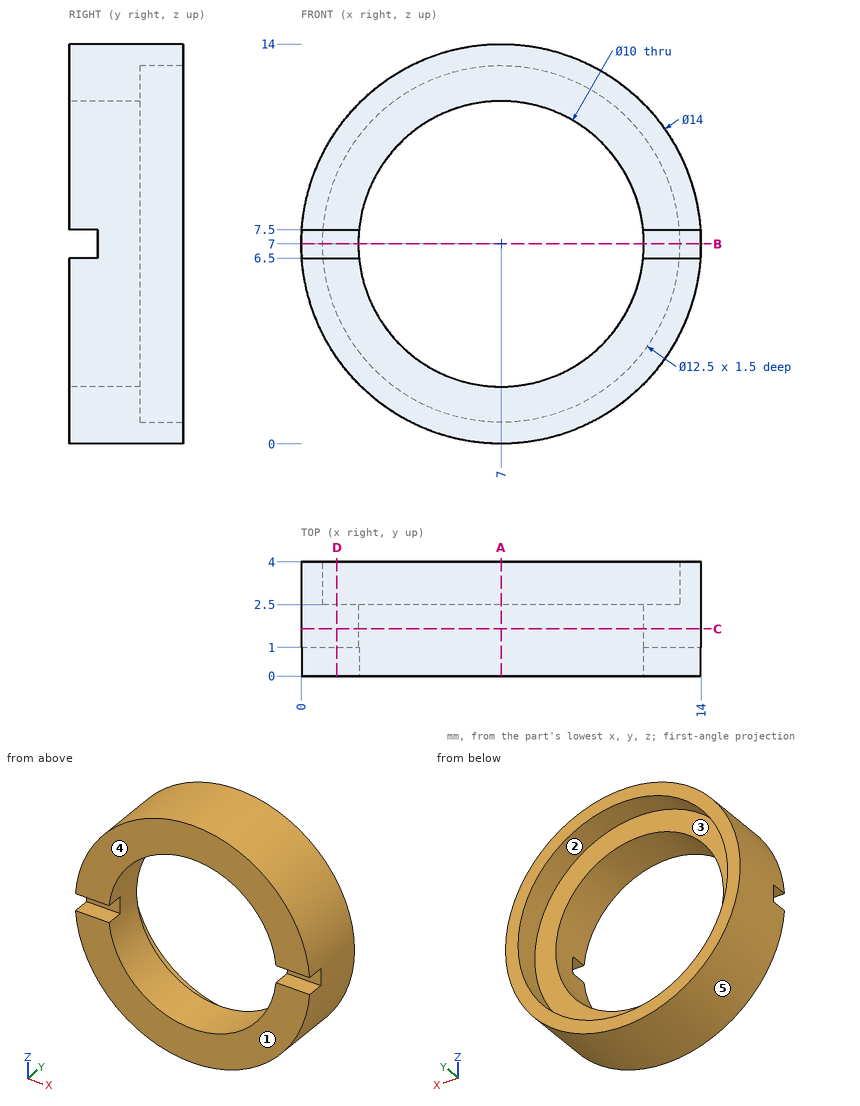
The drawing under review shows one solid part. Ordinate dimensions are in mm from its lowest x, y, z. A direction names the side the tool comes from. Coordinates: 2 decimals unless noted, no trailing zeros. Loops run counter-clockwise (first coordinate to the right, second up) from the corner with the lowest first, then second, coordinate; pieces in that order, holes last.
Item 1: Draft analysis for pull direction Z (two halves, no side actions). For the marked faces 3, 4 and 5, state which applies: pulls with the +Z half, pulls with the -Z half, needs draft (parallel to the pull), parting line crosses it, or undercut.
Completed:
face 3: undercut
face 4: needs draft
face 5: parting line crosses it
Item 2: For the marked faces 1 and 2, list the 3-axis set-ups (+Z, -Z, +X, -X, +Y, -Y) from which the entire face can be reached by the end or side of a thin tool; tool diameter is ignored.
Completed:
face 1: +Z, -Z, +X, -X, -Y
face 2: +Y
Item 3: Wall thickness on L1, parallel to X at y = 3.1, z = 7; L2, parallel to X at y = 1.3, z = 7; L3, parallel to Y at x = 1.25, z = 7.25: over which ranges is each line inside the solid? List them lowest first.
Completed:
L1: x = 0 to 0.75, 13.25 to 14
L2: x = 0 to 2, 12 to 14
L3: y = 1 to 2.5
Item 4: Add section D-D (x = 1.25). Write out the cut boundary in (y, z).
Completed:
outline: (0, 3.01) - (4, 3.01) - (4, 4.55) - (2.5, 4.55) - (2.5, 9.45) - (4, 9.45) - (4, 10.99) - (0, 10.99) - (0, 7.5) - (1, 7.5) - (1, 6.5) - (0, 6.5) - close
Item 5: Clearance check with flat-ended pins moving along their axes: pin 1 (0.5 mm diameter, centred on x = 13.5, z = 7, fed in from -Y); pin 2 (0.8 mm diameter, centred on x = 12.5, y = 0.5, fed in from -Z); pin 3 (0.8 mm diameter, centred on x = 1, y = 0.5, fed in from +Z); pin 4 (4 mm diameter, centred on x = 9, z = 11, fed in from -Y). State where each tip first meets the part, or that it passes through.
Completed:
pin 1: stops at y = 1
pin 2: stops at z = 2.21
pin 3: stops at z = 11.2
pin 4: stops at y = 0
Item 6: Add section C-C (y = 1.65). Write out the cut boundary in (x, z), and give its area (3 significant figures).
Completed:
outline: circle Ø14 at (7, 7); hole circle Ø10 at (7, 7)
area: 75.4 mm2
Item 7: Add section B-B (z = 7). Write out the cut boundary in (x, y), and give its area (3 significant figures).
Completed:
outline: (0, 1) - (2, 1) - (2, 2.5) - (0.75, 2.5) - (0.75, 4) - (0, 4) - close; (12, 1) - (14, 1) - (14, 4) - (13.25, 4) - (13.25, 2.5) - (12, 2.5) - close
area: 8.25 mm2
Item 8: Add section A-A (x = 7). Write out the cut boundary in (y, z), and give its area (4 significant figures).
Completed:
outline: (0, 0) - (4, 0) - (4, 0.75) - (2.5, 0.75) - (2.5, 2) - (0, 2) - close; (0, 12) - (2.5, 12) - (2.5, 13.25) - (4, 13.25) - (4, 14) - (0, 14) - close
area: 12.25 mm2
